from build123d import *

# Parameters (mm, degrees)
F1_DEPTH = 7
F2_R     = 1


with BuildPart() as f1:
    # F0 (on Front) → F1 (new body)
    with BuildSketch(Plane.XZ):
        with BuildLine():
            Line((4, 9.123475), (-4, 9.123475))
            Line((-4, 9.123475), (-4, 5.123475))
            ThreePointArc((-4, 5.123475), (0, 6.5), (4, 5.123475))
            Line((4, 5.123475), (4, 9.123475))
        make_face()
    extrude(amount=F1_DEPTH)

    # F2
    f2_edges = [f1.edges().sort_by_distance(p)[0] for p in [
        (-4, -7, 7.123475),
        (4, -7, 7.123475),
        (4, 0, 7.123475),
        (-4, 0, 7.123475),
        (4, -3.5, 9.123475),
        (-4, -3.5, 9.123475),
        (0, 0, 9.123475),
        (0, -7, 9.123475),
    ]]
    fillet(f2_edges, radius=F2_R)


solid = f1.part
Design review of the part built by this model. Coordinates are the model's own, in mm. Coordinates: 2 decimals unless noted, no trailing zeros. Loops run counter-clockwise (first coordinate to the right, second up) from the corner with the lowest first, then second, coordinate; pieces in that order, holes last. Notation, with made-up numbers: (73.25, 15.5) -> (123.25, 15.5) arc R22 cw to (123.25, 26.5) -> close; hole circle Ø7 at (-34, -12.5). An arc over 180 degrees is marked (long way). Use a Markdown table: item, result. Add a question column.
Item 1: We need section B-B, the plane z = 6.1. Write out the cut boundary in (x, y) (3 decimals).
Item 2: The part is to be moulded in two halves that separate along X. For faces 1 (the flat face through (0, -3, 9.123)), 2 (the flat face through (-4, -3, 7)), 3 (the cylindrical face through (3.715, -6.699, 6.644)), 4 (the cylindrical face through (-0.1, -3.5, 6.5)), say which applies: +X half, -X half, draft (parallel to the pull), parting line (faces both ways), or undercut.
Item 3: We need section A-A, the plane z = 7.8. Write out the cut boundary in (x, y).
Item 4: We need section D-D, the plane x = 0. Write out the cut boundary in (y, z), and give its area (3 significant figures).
Item 5: We need section C-C, the plane y = -5.5. Write out the cut boundary in (x, z).
Item 6: Wall thickness on L1, parallel to X at y = -3.5, z = 5.55; L2, parallel to Z at x = -3, y = -2.25; L3, parallel to Z at x = -3.25, y = -1.5: over which ranges is each line inside the solid? List them lowest first. Write a range as from..to.
Numbers:
| question | item | result |
|---|---|---|
| 1 | outline | (-4, -6) arc R1 ccw to (-3, -7) -> (-2.245, -7) -> (-2.245, 0) -> (-3, 0) arc R1 ccw to (-4, -1) -> close; (2.245, -7) -> (3, -7) arc R1 ccw to (4, -6) -> (4, -1) arc R1 ccw to (3, 0) -> (2.245, 0) -> close |
| 2 | face 1 | draft |
| 2 | face 2 | -X half |
| 2 | face 3 | +X half |
| 2 | face 4 | undercut |
| 3 | outline | (-4, -6) arc R1 ccw to (-3, -7) -> (3, -7) arc R1 ccw to (4, -6) -> (4, -1) arc R1 ccw to (3, 0) -> (-3, 0) arc R1 ccw to (-4, -1) -> close |
| 4 | outline | (-7, 6.5) -> (0, 6.5) -> (0, 8.12) arc R1 ccw to (-1, 9.12) -> (-6, 9.12) arc R1 ccw to (-7, 8.12) -> close |
| 4 | area | 17.9 mm^2 |
| 5 | outline | (-4, 5.12) arc R6.5 cw to (4, 5.12) -> (4, 8.12) arc R1 ccw to (3, 9.12) -> (-3, 9.12) arc R1 ccw to (-4, 8.12) -> close |
| 6 | L1 | x = -4..-3.38, 3.38..4 |
| 6 | L2 | z = 5.77..9.12 |
| 6 | L3 | z = 5.63..9.09 |
